```python
from build123d import *

# Parameters (mm, degrees)
SKETCH1_W                = 300
SKETCH1_H                = 150
BOSS_EXTRUDE1_DEPTH      = 10
SKETCH2_R                = 12.5
CUT_EXTRUDE1_DEPTH       = 169.002976164
M4_CLEARANCE_HOLE1_D     = 4.5
M4_CLEARANCE_HOLE1_DEPTH = 21
M4_CLEARANCE_HOLE1_TIP   = 1.351936393
SKETCH5_R                = 5
CUT_EXTRUDE2_DEPTH       = 169.002976164
SKETCH6_R                = 11
CUT_EXTRUDE3_DEPTH       = 7.2


with BuildPart() as part:
    # Sketch1 → Boss-Extrude1 (new body)
    with BuildSketch(Plane.XY):
        Rectangle(SKETCH1_W, SKETCH1_H)
    extrude(amount=BOSS_EXTRUDE1_DEPTH)

    # Sketch2 → Cut-Extrude1 (cut, through all)
    with BuildSketch(Plane(origin=(0, 0, 0), x_dir=(-1, 0, 0), z_dir=(0, 0, -1))):
        with Locations((0, -51)):
            Circle(SKETCH2_R)
    extrude(amount=-CUT_EXTRUDE1_DEPTH, mode=Mode.SUBTRACT)

    # M4 Clearance Hole1
    with Locations(Plane.XY.offset(10)):
        with Locations((-15.5, -35.5), (15.5, -35.5), (15.5, -66.5), (-15.5, -66.5)):
            Hole(M4_CLEARANCE_HOLE1_D / 2, depth=M4_CLEARANCE_HOLE1_DEPTH)
            with Locations((0, 0, -(M4_CLEARANCE_HOLE1_DEPTH + M4_CLEARANCE_HOLE1_TIP / 2))):  # 118° drill point
                Cone(0, M4_CLEARANCE_HOLE1_D / 2, M4_CLEARANCE_HOLE1_TIP, mode=Mode.SUBTRACT)

    # Sketch5 → Cut-Extrude2 (cut, through all)
    with BuildSketch(Plane.XY.offset(10)):
        with Locations((27.013718503, -25)):
            Circle(SKETCH5_R)
    cut_extrude2 = extrude(amount=-CUT_EXTRUDE2_DEPTH, mode=Mode.SUBTRACT)

    # Mirror1: Cut-Extrude2 across plane
    add(cut_extrude2.mirror(Plane(origin=(0, 0, 0), x_dir=(0, 0, 1), z_dir=(1, 0, 0))), mode=Mode.SUBTRACT)

    # Sketch6 → Cut-Extrude3 (cut)
    with BuildSketch(Plane(origin=(0, 0, 0), x_dir=(-1, 0, 0), z_dir=(0, 0, -1))):
        with Locations((-27.013718503, -25)):
            Circle(SKETCH6_R)
        with Locations((27.013718503, -25)):
            Circle(SKETCH6_R)
    extrude(amount=-CUT_EXTRUDE3_DEPTH, mode=Mode.SUBTRACT)


solid = part.part
```
Work out the finished part from the listing and answer in its coordinate system (mm). A direction names the side the tool comes from. Round coordinates to 2 decimals unless told otherwise and drop trailing zeros. Write each loop counter-clockwise with the first axis right and the second up, starting at its lowest first coordinate (ties: lowest second). Pieces come first, ordered by that corner, then holes. Notation, with made-up numbers: (8.5, -35.5) -> (45.5, -35.5) arc R31 ccw to (45.5, -11.5) -> close; hole circle Ø6 at (4, 54). An arc over 180 degrees is marked (long way). Write each question's results on one line, items separated by ' | '.
Q1. Section B-B, the plane z = 3.5 is taken. Write down the section's boundary in (x, y), then the cut area to 3 significant figures.
Data:
outline: (-150, -75) -> (150, -75) -> (150, 75) -> (-150, 75) -> close; hole circle Ø22 at (-27.01, -25); hole circle Ø4.5 at (-15.5, -66.5); hole circle Ø4.5 at (-15.5, -35.5); hole circle Ø25 at (0, -51); hole circle Ø4.5 at (15.5, -66.5); hole circle Ø4.5 at (15.5, -35.5); hole circle Ø22 at (27.01, -25) | area: 43,700 mm^2
Q2. Section A-A, the plane x = 0 is taken. Write down the section's boundary in (y, z).
Data:
outline: (-75, 0) -> (-63.5, 0) -> (-63.5, 10) -> (-75, 10) -> close; (-38.5, 0) -> (75, 0) -> (75, 10) -> (-38.5, 10) -> close
Q3. Straight lines are drawn through the part: line 1 along Y through (x, z) = (-15.5, 7); line 2 along X through (y, z) = (-24, 1.75); line 3 along X through (y, z) = (-37, 2.5). For each, find the intervals that lie inside material, in ascending order. Write a range as [from, to].
Data:
line 1: [-75, -68.75], [-64.25, -37.75], [-33.25, 75] | line 2: [-150, -37.97], [-16.06, 16.06], [37.97, 150] | line 3: [-150, -17.18], [-13.82, 13.82], [17.18, 150]
Q4. Determine the mould class of faces 1 (the cylindrical face through (-24.63, -35.74, 3.55)), 2 (the flat face through (-2, -75, 5)), 3 (the flat face through (-150, -1, 5)) for opening direction Y: released by +Y, released by -Y, zero draft, split by the parting line, or undercut.
Data:
face 1: undercut | face 2: released by -Y | face 3: zero draft
Q5. Which of the six approach directions +Z, -Z, +X, -X, +Y, -Y give full straight-line access (tool end or side, diameter ignored) to faces 4 (the flat face through (22, -27, 7.2)), 5 (the cylindrical face through (2.71, -63.203, 4.93))?
Data:
face 4: -Z | face 5: +Z, -Z
